from build123d import *

# Parameters (mm, degrees)
BOSS_EXTRUDE1_DEPTH = 1.6
SKETCH2_W           = 17
SKETCH2_H           = 12
BOSS_EXTRUDE2_DEPTH = 1.61
SKETCH3_W           = 14
SKETCH3_H           = 2.4
SKETCH3_W_2         = 13.6
SKETCH3_H_2         = 2
SKETCH3_R           = 0.6
SKETCH3_R_2         = 0.4
BOSS_EXTRUDE3_DEPTH = 1.62
SKETCH3_3_R         = 0.4
CUT_EXTRUDE1_DEPTH  = 2.62
BOSS_EXTRUDE4_START = 1.61
SKETCH4_W           = 3.8
SKETCH4_H           = 5
BOSS_EXTRUDE4_DEPTH = 2
BOSS_EXTRUDE5_START = 1.61
SKETCH5_W           = 2
SKETCH5_H           = 1.2
BOSS_EXTRUDE5_DEPTH = 1
CHAMFER1_SIZE       = 0.3
SKETCH8_W           = 27
SKETCH8_H           = 26
SKETCH8_W_2         = 17
SKETCH8_H_2         = 16
CUT_EXTRUDE9_DEPTH  = 3
SKETCH9_W           = 17
SKETCH9_H           = 3
CUT_EXTRUDE11_DEPTH = 2


with BuildPart() as part:
    # Sketch1 → Boss-Extrude1 (new body)
    with BuildSketch(Plane.XY):
        Polygon((-11.5, 9.5), (-9.5, 11.5), (9.5, 11.5), (11.5, 9.5), (11.5, -9.5), (9.5, -11.5), (-9.5, -11.5), (-11.5, -9.5), align=None)
    extrude(amount=BOSS_EXTRUDE1_DEPTH)

    # Sketch2 → Boss-Extrude2 (add)
    with BuildSketch(Plane.XY):
        Rectangle(SKETCH2_W, SKETCH2_H)
    extrude(amount=BOSS_EXTRUDE2_DEPTH)

    # Sketch3 → Boss-Extrude3 (add)
    with BuildSketch(Plane.XY):
        with Locations((0, -6.5)):
            Rectangle(SKETCH3_W, SKETCH3_H)
        with Locations((0, -6.5)):
            Rectangle(SKETCH3_W_2, SKETCH3_H_2, mode=Mode.SUBTRACT)
        with Locations(Location((-5.08, -6.5, 0), (0, 0, 123.557309762))):
            Circle(SKETCH3_R)
        with Locations((-5.08, -6.5)):
            Circle(SKETCH3_R_2, mode=Mode.SUBTRACT)
        with Locations(Location((-2.54, -6.5, 0), (0, 0, 123.557309762))):
            Circle(SKETCH3_R)
        with Locations((-2.54, -6.5)):
            Circle(SKETCH3_R_2, mode=Mode.SUBTRACT)
        with Locations(Location((0, -6.5, 0), (0, 0, 123.557309762))):
            Circle(SKETCH3_R)
        with Locations((0, -6.5)):
            Circle(SKETCH3_R_2, mode=Mode.SUBTRACT)
        with Locations(Location((5.08, -6.5, 0), (0, 0, 123.557309762))):
            Circle(SKETCH3_R)
        with Locations((5.08, -6.5)):
            Circle(SKETCH3_R_2, mode=Mode.SUBTRACT)
        with Locations(Location((2.54, -6.5, 0), (0, 0, 123.557309762))):
            Circle(SKETCH3_R)
        with Locations((2.54, -6.5)):
            Circle(SKETCH3_R_2, mode=Mode.SUBTRACT)
    extrude(amount=BOSS_EXTRUDE3_DEPTH)

    # Sketch3<3> → Cut-Extrude1 (cut)
    with BuildSketch(Plane.XY):
        with Locations((-5.08, -6.5)):
            Circle(SKETCH3_3_R)
        with Locations((-2.54, -6.5)):
            Circle(SKETCH3_3_R)
        with Locations((0, -6.5)):
            Circle(SKETCH3_3_R)
        with Locations((2.54, -6.5)):
            Circle(SKETCH3_3_R)
        with Locations((5.08, -6.5)):
            Circle(SKETCH3_3_R)
    extrude(amount=CUT_EXTRUDE1_DEPTH, mode=Mode.SUBTRACT)

    # Sketch4 → Boss-Extrude4 (add)
    with BuildSketch(Plane.XY.offset(BOSS_EXTRUDE4_START)):
        Rectangle(SKETCH4_W, SKETCH4_H)
    extrude(amount=BOSS_EXTRUDE4_DEPTH)

    # Sketch5 → Boss-Extrude5 (add)
    with BuildSketch(Plane.XY.offset(BOSS_EXTRUDE5_START)):
        with Locations((-4.500129294, -1.9)):
            Rectangle(SKETCH5_W, SKETCH5_H)
        with Locations((-4.5, 0.5)):
            Rectangle(SKETCH5_W, SKETCH5_H)
        with Locations((4.5, -1.9)):
            Rectangle(SKETCH5_W, SKETCH5_H)
    extrude(amount=BOSS_EXTRUDE5_DEPTH)

    # Chamfer1
    chamfer1_edges = [part.edges().sort_by_distance(p)[0] for p in [
        (1.9, 0, 3.61),
        (0, 2.5, 3.61),
        (-1.9, 0, 3.61),
        (0, -2.5, 3.61),
    ]]
    chamfer(chamfer1_edges, length=CHAMFER1_SIZE)

    # Sketch8 → Cut-Extrude9 (cut)
    with BuildSketch(Plane.XY):
        Rectangle(SKETCH8_W, SKETCH8_H)
        Rectangle(SKETCH8_W_2, SKETCH8_H_2, mode=Mode.SUBTRACT)
    extrude(amount=CUT_EXTRUDE9_DEPTH, mode=Mode.SUBTRACT)

    # Sketch9 → Cut-Extrude11 (cut)
    with BuildSketch(Plane.XY):
        with Locations((0, 6.5)):
            Rectangle(SKETCH9_W, SKETCH9_H)
    extrude(amount=CUT_EXTRUDE11_DEPTH, mode=Mode.SUBTRACT)


solid = part.part
Verification items for the finished model (mm, model axes). A direction names the side the tool comes from. Coordinates: 2 decimals unless noted, no trailing zeros. Write each loop counter-clockwise with the first axis right and the second up, starting at its lowest first coordinate (ties: lowest second). Pieces come first, ordered by that corner, then holes. Notation, with made-up numbers: M -14.5,45.5 L 6.5,45.5 A8 ccw 6.5,59.5 Z; hole C -22,42 d11. An arc over 180 degrees is marked long. Use a Markdown table: item, result.
Q1. Thickness scan on line 1 (Y direction, x = 5.08, z = 1.15); line 2 (Z direction, x = 5.5, y = 3); line 3 (Y direction, x = -2.25, z = 1.25). Record the ranges inside material, lowest first.
Reply:
| item | result |
|---|---|
| line 1 | y = -8 to -6.9, -6.1 to 5 |
| line 2 | z = 0 to 1.61 |
| line 3 | y = -8 to -6.78, -6.22 to 5 |
Q2. Sectioned sample at B-B, the plane y = -2. Record the boundary of the cut face in (x, z).
Reply:
| item | result |
|---|---|
| outline | M -8.5,0 L 8.5,0 L 8.5,1.61 L 5.5,1.61 L 5.5,2.61 L 3.5,2.61 L 3.5,1.61 L 1.9,1.61 L 1.9,3.31 L 1.6,3.61 L -1.6,3.61 L -1.9,3.31 L -1.9,1.61 L -3.5,1.61 L -3.5,2.61 L -5.5,2.61 L -5.5,1.61 L -8.5,1.61 Z |
Q3. Draft check along X on faces 4 (the face through (4, -2, 2.61)), 5 (the face through (5.5, -2, 2)), 6 (the face through (-1, -7, 1.6)). Enter one of: +X half, -X half, draft (parallel to the pull), parting line (faces both ways), or undercut.
Reply:
| item | result |
|---|---|
| face 4 | draft |
| face 5 | +X half |
| face 6 | undercut |
Q4. Sectioned sample at D-D, the plane y = -6.5. Count the separate pieces of the cut face and the enclosed holes in it, plus the area to 3 significant figures.
Reply:
| item | result |
|---|---|
| separate pieces | 6 |
| enclosed holes | 0 |
| area | 20.8 mm² |
Q5. Set-up check for faces 1 (the face through (-5, -1.3, 2)), 2 (the face through (-3.5, -2, 2)), 3 (the face through (0, 2.5, 2)): record each of +Z, -Z, +X, -X, +Y, -Y from which the full face is reachable in a straight line by a thin tool's end or side.
Reply:
| item | result |
|---|---|
| face 1 | +Z, -X |
| face 2 | +Z, +Y, -Y |
| face 3 | +Z, +X, -X, +Y |
Q6. Go/stop test with flat-tipped pins: P1, Ø0.9, axis at x = -0.5, z = 2, coming from the -Y side; P2, Ø0.6, axis at x = 4.5, y = -2, coming from the +Z side; P3, Ø0.7, axis at x = -1, y = -7, coming from the +Z side. Record where each tip stops, or that it passes through.
Reply:
| item | result |
|---|---|
| P1 | stops at y = -8 |
| P2 | stops at z = 2.61 |
| P3 | stops at z = 1.6 |
